Can you work these out from the model? Positions are in its coordinate system, mm. A direction names the side the tool comes from. Coordinates: 2 decimals unless noted, no trailing zeros. Order: outer loops, then holes, each group sorted by start corner. A loop starts at its lowest first (then second) coordinate and runs counter-clockwise, first axis right, second up. Notation, with made-up numbers: (65.25, 16.5) -> (113.25, 16.5) arc R23 cw to (113.25, 51.5) -> close; hole circle Ø1 at (39.5, 51.25). An arc over 180 degrees is marked (long way). Answer as a JSON object with one key per item and string values. Group by question number.
(1) I want a section at A-A, the plane y = 0. List the corners of the cut face in (x, z) for me.
(2) For pin 1 (7 mm diameter, centred on x = 29.9, y = -35, fed in from +Z); pin 2 (2 mm diameter, centred on x = -38.5, z = 0.5, fed in from -Y); pin 3 (5.5 mm diameter, centred on x = -38.5, y = 1.5, fed in from +Z); pin 4 (2 mm diameter, centred on x = 39, z = 1, fed in from +Y), each with a flat end and sliding along its axis, tell me the tip position at first contact or that it passes through.
(3) I need wall thicknesses on line 1 (X direction, y = 35, z = 3.7); line 2 (Y direction, x = -29.9, z = 3); line 3 (Y direction, x = 0, z = 2.8). Which ranges of each line are inside material? Lowest first, please.
(4) I want a section at D-D, the plane y = -35. List the corners of the cut face in (x, z) for me.
(5) Which directions (+Z, -Z, +X, -X, +Y, -Y) give clear straight access to the entire face, cutting with the end or side of a thin tool? Please do faces 1 (the flat face through (-38, -29.9, 1)), 2 (the flat face through (38, 29.9, 1)), 3 (the flat face through (37, 0, 2.8)).
(6) I want a section at C-C, the plane z = 3.6. List the corners of the cut face in (x, y) for me, plus the area to 3 significant figures.
(7) I want a section at B-B, the plane x = 29.9. List the corners of the cut face in (y, z) for me, plus the area to 3 significant figures.
Autodesk Inventor part; units mm, degrees
ref_plane "YZ Plane" through (0, 0, 0) normal (1, 0, 0) x (0, 1, 0)
ref_plane "XZ Plane" through (0, 0, 0) normal (0, 1, 0) x (-1, 0, 0)
ref_plane "XY Plane" through (0, 0, 0) normal (0, 0, 1) x (1, 0, 0)
sketch "スケッチ1" plane through (0, 0, 0) normal (0, 0, 1) x (1, 0, 0)
  circle A0 centre (0, 0) radius 27.6
  line L0 (-40, 40) -> (40, 40)
  line L1 (40, 40) -> (40, -40)
  line L2 (40, -40) -> (-40, -40)
  line L3 (-40, -40) -> (-40, 40)
  dimension "d0" = 55.2
  dimension "d1" = 40
  dimension "d2" = 80
  dimension "d3" = 80
  dimension "d4" = 40
extrude "押し出し1" add sketch "スケッチ1" along normal blind 5
sketch "スケッチ3" plane through (0, 0, 5) normal (0, 0, 1) x (1, 0, 0)
  line L0 (40, -40) -> (-40, -40)
  line L1 (-40, 40) -> (-34.9, 40)
  line L2 (-34.9, 40) -> (-34.9, -40)
  line L3 (-34.9, -40) -> (-40, -40)
  line L4 (-40, -40) -> (-40, 40)
  line L5 (40, 40) -> (34.9, 40)
  line L6 (34.9, 40) -> (34.9, -40)
  line L7 (34.9, -40) -> (40, -40)
  line L8 (40, -40) -> (40, 40)
  dimension "d17" = 5.1
  dimension "d18" = 5.1
extrude "押し出し3" cut sketch "スケッチ3" against normal blind 2.2
sketch "スケッチ4" plane through (0, 0, 0) normal (0, 0, -1) x (-1, 0, 0)
  line L0 (-40, 40) -> (-34.9, 40)
  line L1 (-34.9, 40) -> (-34.9, 29.9)
  line L2 (-34.9, 29.9) -> (-40, 29.9)
  line L3 (-40, 29.9) -> (-40, 40)
  line L4 (-40, -40) -> (-34.9, -40)
  line L5 (-34.9, -40) -> (-34.9, -29.9)
  line L6 (-34.9, -29.9) -> (-40, -29.9)
  line L7 (-40, -29.9) -> (-40, -40)
  line L8 (40, 40) -> (34.9, 40)
  line L9 (34.9, 40) -> (34.9, 29.9)
  line L10 (34.9, 29.9) -> (40, 29.9)
  line L11 (40, 29.9) -> (40, 40)
  line L12 (40, -40) -> (34.9, -40)
  line L13 (34.9, -40) -> (34.9, -29.9)
  line L14 (34.9, -29.9) -> (40, -29.9)
  line L15 (40, -29.9) -> (40, -40)
  dimension "d21" = 5.1
  dimension "d22" = 10.1
  dimension "d23" = 10.1
  dimension "d24" = 10.1
  dimension "d25" = 5.1
  dimension "d26" = 5.1
  dimension "d27" = 5.1
  dimension "d28" = 10.1
extrude "押し出し4" cut sketch "スケッチ4" against normal through all
sketch "スケッチ5" plane through (0, 0, 0) normal (0, 0, -1) x (-1, 0, 0)
  line L0 (-40, -29.9) -> (-34.9, -29.9)
  line L1 (-34.9, -29.9) -> (-34.9, -40)
  line L2 (34.9, -40) -> (34.9, -29.9)
  line L3 (34.9, -29.9) -> (40, -29.9)
  line L4 (40, 29.9) -> (34.9, 29.9)
  line L5 (34.9, 29.9) -> (34.9, 40)
  line L6 (-34.9, 40) -> (-34.9, 29.9)
  line L7 (-34.9, 29.9) -> (-40, 29.9)
  point P0 (-35.9, 29.9)
  point P1 (-35.9, -29.9)
  point P2 (35.9, -29.9)
  point P3 (35.9, 29.9)
  dimension "d31" = 1
  dimension "d32" = 1
  dimension "d33" = 1
  dimension "d34" = 1
hole "Hole1" at (35.9, 29.9, 0) at (35.9, -29.9, 0) at (-35.9, -29.9, 0) at (-35.9, 29.9, 0) direction (0, 0, 1) diameter 2 end through all
sketch "スケッチ6" plane through (0, 0, 0) normal (0, 0, -1) x (-1, 0, 0)
  line L0 (34.9, 29.9) -> (34.9, 40)
  line L1 (34.9, 40) -> (-34.9, 40)
  line L2 (-34.9, 40) -> (-34.9, 29.9)
  line L3 (-34.9, -29.9) -> (-34.9, -40)
  line L4 (-34.9, -40) -> (34.9, -40)
  line L5 (34.9, -40) -> (34.9, -29.9)
  point P0 (-29.9, 35)
  point P1 (-29.9, -35)
  point P2 (29.9, -35)
  point P3 (29.9, 35)
  dimension "d42" = 5
  dimension "d43" = 5
  dimension "d44" = 5
  dimension "d45" = 5
  dimension "d46" = 5
  dimension "d47" = 5
  dimension "d48" = 5
  dimension "d49" = 5
hole "Hole2" at (29.9, 35, 0) at (29.9, -35, 0) at (-29.9, -35, 0) at (-29.9, 35, 0) direction (0, 0, 1) diameter 6 end through all
equation "\"d1\" = 0.5 * d2"
equation "\"d3\" = d2"
equation "\"d18\" = d17"
equation "\"d23\" = d22"
equation "\"d25\" = d21"
equation "\"d26\" = d21"
equation "\"d27\" = d21"
equation "\"d28\" = d22"
properties part number "JointA2"
Computed values:
{
 "1": {"outline": "(-40, 0) -> (-27.6, 0) -> (-27.6, 5) -> (-34.9, 5) -> (-34.9, 2.8) -> (-40, 2.8) -> close; (27.6, 0) -> (40, 0) -> (40, 2.8) -> (34.9, 2.8) -> (34.9, 5) -> (27.6, 5) -> close"},
 "2": {"pin 1": "stops at z = 5", "pin 2": "stops at y = -29.9", "pin 3": "stops at z = 2.8", "pin 4": "stops at y = 29.9"},
 "3": {"line 1": "x = -34.9 to -32.9, -26.9 to 26.9, 32.9 to 34.9", "line 2": "y = -40 to -38, -32 to 32, 38 to 40", "line 3": "y = -40 to -27.6, 27.6 to 40"},
 "4": {"outline": "(-34.9, 0) -> (-32.9, 0) -> (-32.9, 5) -> (-34.9, 5) -> close; (-26.9, 0) -> (26.9, 0) -> (26.9, 5) -> (-26.9, 5) -> close; (32.9, 0) -> (34.9, 0) -> (34.9, 5) -> (32.9, 5) -> close"},
 "5": {"face 1": "+Z, -Z, -X, -Y", "face 2": "+Z, -Z, +X, +Y", "face 3": "+Z, +X, +Y, -Y"},
 "6": {"outline": "(-34.9, -40) -> (34.9, -40) -> (34.9, 40) -> (-34.9, 40) -> close; hole circle Ø6 at (-29.9, -35); hole circle Ø6 at (-29.9, 35); hole circle Ø55.2 at (0, 0); hole circle Ø6 at (29.9, -35); hole circle Ø6 at (29.9, 35)", "area": "3,080 mm2"},
 "7": {"outline": "(-40, 0) -> (-38, 0) -> (-38, 5) -> (-40, 5) -> close; (-32, 0) -> (32, 0) -> (32, 5) -> (-32, 5) -> close; (38, 0) -> (40, 0) -> (40, 5) -> (38, 5) -> close", "area": "340 mm2"}
}
